Study the drawing (mm; zero at the part's minimum x, y, z) and answer. A direction names the side the tool comes from. Round coordinates to 2 decimals unless told otherwise and drop trailing zeros. Order: outer loops, then holes, each group sorted by start corner. A loop starts at its lowest first (then second) coordinate and runs counter-clockwise, first axis right, second up. Notation, with made-up numbers: (46, -37.75) -> (82, -37.75) arc R25 cw to (82, -1.75) -> close; hole circle Ø5 at (89.5, 15). An arc over 180 degrees is marked (long way). Answer in a Markdown table with one row per item. Add a question column.
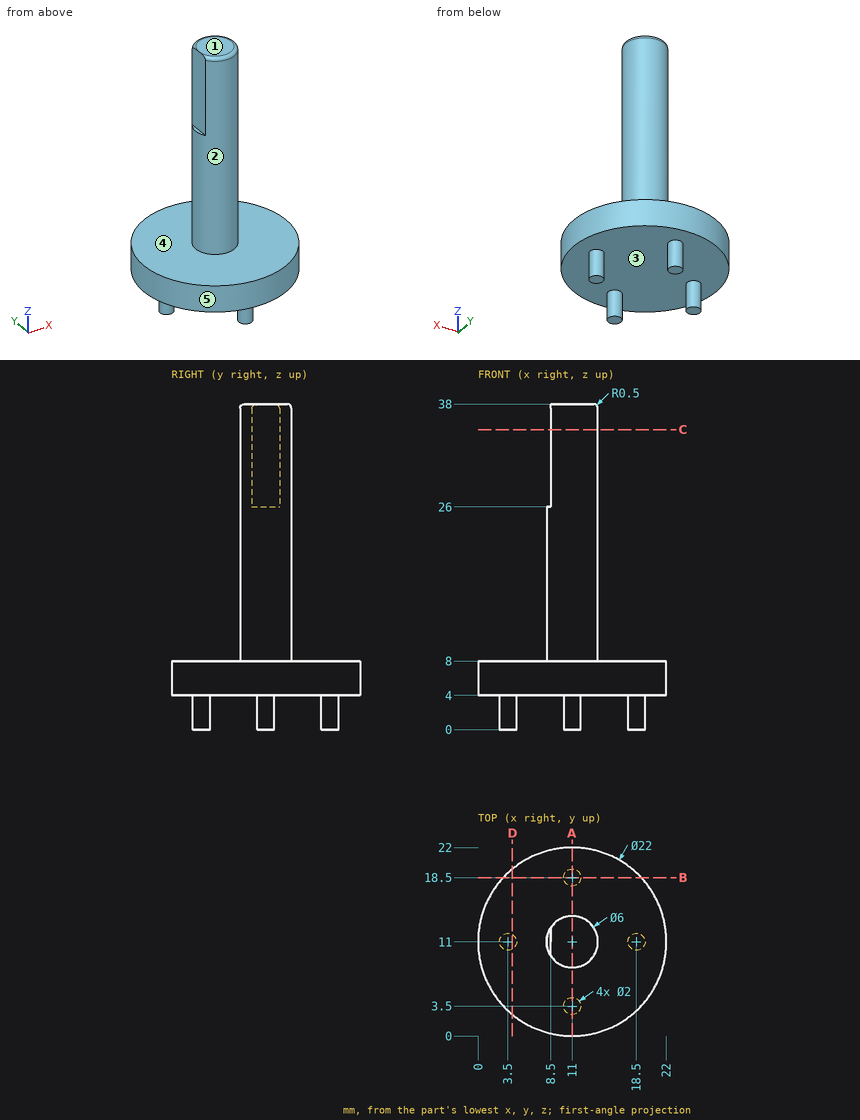
Item 1: For a pull along Z with two mould halves and no side action, classify the marked faces 1, 2 and 3 as released by +Z, released by -Z, zero draft, split by the parting line, or undercut.
Item 2: Find the intervals of material crossed by probe 1 along Z at (x, y) = (13, 4.5); probe 2 along Y at (x, z) = (20, 5.5); probe 3 along Y at (x, z) = (10.5, 3), in increasing order. Write a range as [from, to].
Item 3: The part is cut by section D-D, the plane x = 4. Give the vertices of the cut face in (y, z).
Item 4: A tool of negligible diameter and unlimited length cuts with its end or side. For the marked faces 4 and 5, from which of +Z, -Z, +X, -X, +Y, -Y can it reach the whole face along a straight path? Write none if from no direction.
Item 5: The part is cut by section B-B, the plane y = 18.5. Give the vertices of the cut face in (x, z), and give its area (3 significant figures).
Item 6: The part is cut by section A-A, the plane x = 11. Give the vertices of the cut face in (y, z), and give its area (3 significant figures).
Item 7: The part is cut by section C-C, the plane z = 35. Give the vertices of the cut face in (x, y), and give its area (3 significant figures).
Item 8: Flat-ended cylindrical pins translate along their axes: P1, Ø5, axis at x = 16, y = 17.5, coming from the -Z side; P2, Ø1, axis at x = 10, y = 3.5, coming from the +Z side; P3, Ø8, axis at x = 17.5, z = 15, coming from the +Y side. Find the tip coordinate at first contact, or state that the pin passes through.
Resolved:
| question | item | result |
|---|---|---|
| 1 | face 1 | released by +Z |
| 1 | face 2 | zero draft |
| 1 | face 3 | released by -Z |
| 2 | probe 1 | [4, 8] |
| 2 | probe 2 | [4.68, 17.32] |
| 2 | probe 3 | [2.63, 4.37], [17.63, 19.37] |
| 3 | outline | (2.51, 4) -> (10.13, 4) -> (10.13, 0) -> (11.87, 0) -> (11.87, 4) -> (19.49, 4) -> (19.49, 8) -> (2.51, 8) -> close |
| 4 | face 4 | +Z |
| 4 | face 5 | +Z, -Z |
| 5 | outline | (2.95, 4) -> (10, 4) -> (10, 0) -> (12, 0) -> (12, 4) -> (19.05, 4) -> (19.05, 8) -> (2.95, 8) -> close |
| 5 | area | 72.4 mm2 |
| 6 | outline | (0, 4) -> (2.5, 4) -> (2.5, 0) -> (4.5, 0) -> (4.5, 4) -> (17.5, 4) -> (17.5, 0) -> (19.5, 0) -> (19.5, 4) -> (22, 4) -> (22, 8) -> (14, 8) -> (14, 37.5) arc R0.5 ccw to (13.5, 38) -> (8.5, 38) arc R0.5 ccw to (8, 37.5) -> (8, 8) -> (0, 8) -> close |
| 6 | area | 284 mm2 |
| 7 | outline | (8.5, 9.34) arc R3 ccw (long way) to (8.5, 12.66) -> close |
| 7 | area | 27.1 mm2 |
| 8 | P1 | z = 4 |
| 8 | P2 | z = 8 |
| 8 | P3 | y = 12.66 |
